Design review of the part built by this model. Coordinates are the model's own, in mm. A direction names the side the tool comes from. Coordinates: 2 decimals unless noted, no trailing zeros. Loops run counter-clockwise (first coordinate to the right, second up) from the corner with the lowest first, then second, coordinate; pieces in that order, holes last. Notation, with made-up numbers: M -5.5,64 L 26.5,64 A24 ccw 26.5,96 Z; hole C 77,-6.5 d10. An arc over 180 degrees is marked long. Put each result on its own line as item: value. Start each with the question number.
(1) The part is to be moulded in two halves that separate along Y. For faces 1 (the cylindrical face through (-2.17, -9.76, 6.41)), 2 (the cylindrical face through (-24.93, -1.08, -26.88)), 3 (the flat face through (-9, 5, 0)), 4 (the flat face through (-24, 15, -2)), say which applies: +Y half, -Y half, draft (parallel to the pull), parting line (faces both ways), or undercut.
(2) For probe 1 along X at (y, z) = (-5.5, -28.5); probe 2 along Z at (x, y) = (-26.5, 0); probe 3 along Y at (x, z) = (0, 4), list the stretches that pass through material, from the lowest coordinate up. Write a range as [from, to].
(3) Clearance check with flat-ended pins moving along their axes: pin 1 (13.5 mm diameter, centred on x = 22, z = -7.5, fed in from +Y); pin 2 (5 mm diameter, centred on x = 25.5, z = -1, fed in from -Y); pin 3 (20 mm diameter, centred on x = 3, y = 6, fed in from -Z). State where each tip first meets the part, or that it passes through.
(4) Take a section at D-D, the plane z = 5. Give the boundary of the cut face in (x, y), then the cut area to 3 significant figures.
(5) Take a section at A-A, the plane z = -14.5. Give the boundary of the cut face in (x, y), then the cut area to 3 significant figures.
(6) Take a section at C-C, the plane y = 0. Give the boundary of the cut face in (x, z).
(7) Take a section at B-B, the plane x = 0. Give the boundary of the cut face in (y, z).
(8) For faces 5 (the flat face through (-24, -15, -2)), 6 (the flat face through (-0.4, -17.5, 10)), 7 (the flat face through (-20, 0, -14)), list the 3-axis set-ups (+Z, -Z, +X, -X, +Y, -Y) from which the entire face can be reached by the end or side of a thin tool; tool diameter is ignored.
```python
from build123d import *

# Parameters (mm, degrees)
F0_R     = 10
F1_DEPTH = 10
F2_R     = 17
F2_R_2   = 10
F3_DEPTH = 3
F4_W     = 10
F4_H     = 30
F5_DEPTH = 37
F6_R     = 5
F7_DEPTH = 60.001


with BuildPart() as f1:
    # F0 (on Top) → F1 (new body)
    with BuildSketch(Plane.XY):
        with BuildLine():
            Line((30, -15), (30, 15))
            Line((30, 15), (13.2287565553, 15))
            ThreePointArc((13.2287565553, 15), (18.2287565553, 8.2287565553), (20, 0))
            ThreePointArc((20, 0), (18.2287565553, -8.2287565553), (13.2287565553, -15))
            Line((13.2287565553, -15), (30, -15))
        make_face()
        with BuildLine():
            ThreePointArc((20, 0), (18.2287565553, 8.2287565553), (13.2287565553, 15))
            Line((13.2287565553, 15), (-13.2287565553, 15))
            ThreePointArc((-13.2287565553, 15), (-20, 0), (-13.2287565553, -15))
            Line((-13.2287565553, -15), (13.2287565553, -15))
            ThreePointArc((13.2287565553, -15), (18.2287565553, -8.2287565553), (20, 0))
        make_face()
        Circle(F0_R, mode=Mode.SUBTRACT)
        with BuildLine():
            Line((-13.2287565553, 15), (13.2287565553, 15))
            ThreePointArc((13.2287565553, 15), (0, 20), (-13.2287565553, 15))
        make_face()
        with BuildLine():
            ThreePointArc((-13.2287565553, -15), (-20, 0), (-13.2287565553, 15))
            Line((-13.2287565553, 15), (-30, 15))
            Line((-30, 15), (-30, -15))
            Line((-30, -15), (-13.2287565553, -15))
        make_face()
        with BuildLine():
            ThreePointArc((-13.2287565553, -15), (0, -20), (13.2287565553, -15))
            Line((13.2287565553, -15), (-13.2287565553, -15))
        make_face()
    extrude(amount=F1_DEPTH)

    # F2 (on face) → F3 (join)
    with BuildSketch(Plane.XY.offset(10)):
        Circle(F2_R)
        Circle(F2_R_2, mode=Mode.SUBTRACT)
    extrude(amount=F3_DEPTH)

    # F4 (on face) → F5 (join)
    with BuildSketch(Plane(origin=(0, 0, 0), x_dir=(1, 0, 0), z_dir=(0, 0, -1))):
        with Locations((-25, 0)):
            Rectangle(F4_W, F4_H)
        with Locations((25, 0)):
            Rectangle(F4_W, F4_H)
    extrude(amount=F5_DEPTH)

    # F6 (on face) → F7 (cut, through all)
    with BuildSketch(Plane.YZ.offset(30)):
        with BuildLine():
            ThreePointArc((0, -37), (-10.6066017409, -32.6066016947), (-15, -21.9999999346))
            Line((-15, -21.9999999346), (-15, -37))
            Line((-15, -37), (0, -37))
        make_face()
        with BuildLine():
            Line((15, -37), (15, -22))
            ThreePointArc((15, -22), (10.6066017178, -32.6066017178), (0, -37))
            Line((0, -37), (15, -37))
        make_face()
        with Locations((0, -22)):
            Circle(F6_R)
    extrude(amount=-F7_DEPTH, mode=Mode.SUBTRACT)


solid = f1.part
```
Computed values:
1. face 1: undercut
1. face 2: undercut
1. face 3: draft
1. face 4: +Y half
2. probe 1: x = [-30, -20], [20, 30]
2. probe 2: z = [-37, -27], [-17, 10]
2. probe 3: y = [-20, -10], [10, 20]
3. pin 1: stops at y = 15
3. pin 2: stops at y = -15
3. pin 3: stops at z = 0
4. outline: M -30,-15 L -13.23,-15 A20 ccw 13.23,-15 L 30,-15 L 30,15 L 13.23,15 A20 ccw -13.23,15 L -30,15 Z; hole C 0,0 d20
4. area: 1,670 mm^2
5. outline: M -30,-15 L -20,-15 L -20,15 L -30,15 Z; M 20,-15 L 30,-15 L 30,15 L 20,15 Z
5. area: 600 mm^2
6. outline: M -30,-37 L -20,-37 L -20,-27 L -30,-27 Z; M -30,-17 L -20,-17 L -20,0 L -10,0 L -10,13 L -17,13 L -17,10 L -30,10 Z; M 10,0 L 20,0 L 20,-17 L 30,-17 L 30,10 L 17,10 L 17,13 L 10,13 Z; M 20,-37 L 30,-37 L 30,-27 L 20,-27 Z
7. outline: M -20,0 L -10,0 L -10,13 L -17,13 L -17,10 L -20,10 Z; M 10,0 L 20,0 L 20,10 L 17,10 L 17,13 L 10,13 Z
8. face 5: +Z, -Z, -X, -Y
8. face 6: +Z
8. face 7: -Z, +Y, -Y
